Geometry check sheet. Reference: the model listing, model coordinates, mm. Round coordinates to 2 decimals unless told otherwise and drop trailing zeros. Write each loop counter-clockwise with the first axis right and the second up, starting at its lowest first coordinate (ties: lowest second). Pieces come first, ordered by that corner, then holes.
Item 1: Cross-section at C-C (z = 5.2). Enter the section's corners in (x, y), then the cut area to 3 significant figures.
Item 2: Cross-section at A-A (y = -30). Enter the section's corners in (x, z).
Item 3: Cross-section at B-B (x = 0). Enter the section's corners in (y, z).
Item 4: Depth check by flat-ended pin: P1, Ø1, axis at x = 3.5, y = -24.5, coming from the -Z side. Enter the tip coordinate at first touch or a pass-through.
Item 5: Draft check along Y on faces 1 (the face through (0, -36, 3)), 2 (the face through (0, 1, 0)), 3 (the face through (-0.521, 33.966, 2.958)). Enter one of: pulls with the +Y half, pulls with the -Y half, needs draft (parallel to the pull), parting line crosses it, or undercut.
Item 6: Scan lines: probe 1 along Y at (x, z) = (0, 1.9); probe 2 along X at (y, z) = (30, 3.2); probe 3 along Y at (x, z) = (-2.75, 4.55). Record each from-to range of solid material in increasing order.
from build123d import *

# Parameters (mm, degrees)
SKETCH_4_W               = 12
SKETCH_4_H               = 72
EXTRUDE_1_DEPTH          = 6
CUT_EXTRUDE_1_DEPTH      = 37.986484018
CUT_EXTRUDE_1_DEPTH_BACK = 37.986484018
SKETCH_5_R               = 4
CHAMFER_1_SIZE           = 1


with BuildPart() as part:
    # ｽｹｯﾁ4 → ﾎﾞｽ - 押し出し1 (new body)
    with BuildSketch(Plane.XY):
        Rectangle(SKETCH_4_W, SKETCH_4_H)
    extrude(amount=EXTRUDE_1_DEPTH)

    # ｽｹｯﾁ5 → ｶｯﾄ - 押し出し1 (cut, two sides: drawn at the far end of the back side and taken through both)
    with BuildSketch(Plane.XY.offset(6).offset(-CUT_EXTRUDE_1_DEPTH_BACK)):
        with Locations((0, 30)):
            Circle(SKETCH_5_R)
        with Locations((0, -30)):
            Circle(SKETCH_5_R)
    extrude(amount=CUT_EXTRUDE_1_DEPTH + CUT_EXTRUDE_1_DEPTH_BACK, mode=Mode.SUBTRACT)

    # 面取り1
    chamfer_1_edges = [part.edges().sort_by_distance(p)[0] for p in [
        (6, -36, 3),
        (-6, -36, 3),
        (-6, 36, 3),
        (6, 36, 3),
    ]]
    chamfer(chamfer_1_edges, length=CHAMFER_1_SIZE)


solid = part.part
Resolved:
1. outline: (-6, -35) - (-5, -36) - (5, -36) - (6, -35) - (6, 35) - (5, 36) - (-5, 36) - (-6, 35) - close; hole circle Ø8 at (0, -30); hole circle Ø8 at (0, 30)
1. area: 761 mm2
2. outline: (-6, 0) - (-4, 0) - (-4, 6) - (-6, 6) - close; (4, 0) - (6, 0) - (6, 6) - (4, 6) - close
3. outline: (-36, 0) - (-34, 0) - (-34, 6) - (-36, 6) - close; (-26, 0) - (26, 0) - (26, 6) - (-26, 6) - close; (34, 0) - (36, 0) - (36, 6) - (34, 6) - close
4. P1: stops at z = 0
5. face 1: pulls with the -Y half
5. face 2: needs draft
5. face 3: undercut
6. probe 1: y = -36 to -34, -26 to 26, 34 to 36
6. probe 2: x = -6 to -4, 4 to 6
6. probe 3: y = -36 to -32.9, -27.1 to 27.1, 32.9 to 36
